Source: CAD feature listing. Evaluate the final solid. Frame: model axes, mm. A direction names the side the tool comes from. Coordinates: 2 decimals unless noted, no trailing zeros. Order: outer loops, then holes, each group sorted by start corner. A loop starts at its lowest first (then second) coordinate and runs counter-clockwise, first axis right, second up. Notation, with made-up numbers: (81.5, 51) - (124.5, 51) arc R20 ccw to (124.5, 68) - close; hole circle Ø7 at (65, 22). An arc over 180 degrees is marked (long way). One line per question, with ' | ' between items. Start each with the question number.
(1) Access query for faces 1 (the flat face through (17.26, 32.27, 22.76)), 2 (the cylindrical face through (16.241, 85.058, -29.11)). Directions: +Z, -Z, +X, -X, +Y, -Y. A direction counts if a zero-diameter tool reaches every point of the face in a straight line with its end or side. Return the directions, or none.
(2) Contact query for flat-ended pins moving along their axis: P1, Ø5, axis at x = 30.5, z = -22, coming from the +Y side; P2, Ø13, axis at y = 22.26, z = 32.96, coming from the -X side; P3, Ø8, axis at x = 16, z = -38.5, coming from the +Y side; P4, Ø9, axis at y = -47.74, z = 32.96, coming from the -X side. Output: stop coordinate, or through.
(3) Section C-C (y = 13.5). Return the cut outline in (x, z).
(4) Section D-D (z = -10.5). Return the cut outline in (x, y).
(5) Section B-B (z = 34.5). Return the cut outline in (x, y).
(6) Draft query along Y for faces 3 (the flat face through (17, -14, 42.956)), 4 (the flat face through (35, 35, 5)), 5 (the flat face through (16.24, 51.94, -0.06)). Return one class per face: +Y half, -Y half, draft (parallel to the pull), parting line (faces both ways), or undercut.
(7) Line query: line 1 along Z through (x, y) = (33.5, 5.5); line 2 along X through (y, z) = (26, 17); line 3 along Y through (x, z) = (3, -10.5). Output: solid intervals per line, ascending.
(8) Section A-A (x = 7.5). Return the cut outline in (y, z).
from build123d import *

# Parameters (mm, degrees)
SKETCH1_R           = 5
BOSS_EXTRUDE1_DEPTH = 2
EXTRUDE_THIN1_DEPTH = 35


# Read off the part's stored shape, not the designer's step: Extrude-Thin1
with BuildPart() as part:
    # Sketch1 → Boss-Extrude1 (new body)
    with BuildSketch(Plane(origin=(0, 0, 0), x_dir=(0, 0, -1), z_dir=(1, 0, 0))):
        with BuildLine():
            Line((49.043932947, -59.7371598), (-44.956067053, -59.7371598))
            Line((-44.956067053, -59.7371598), (-44.956067053, 32.2628402))
            Line((-44.956067053, 32.2628402), (-3.612044261, 36.014733483))
            Line((-3.612044261, 36.014733483), (3.632035406, 67.43070713))
            ThreePointArc((3.632035406, 67.43070713), (28.644544082, 85.115341633), (49.043932947, 62.2628402))
            Line((49.043932947, 62.2628402), (49.043932947, -59.7371598))
        make_face()
        with Locations((37.043932947, 22.2628402)):
            Circle(SKETCH1_R, mode=Mode.SUBTRACT)
        with Locations((37.043932947, -47.7371598)):
            Circle(SKETCH1_R, mode=Mode.SUBTRACT)
        with Locations((-32.956067053, -47.7371598)):
            Circle(SKETCH1_R, mode=Mode.SUBTRACT)
        with Locations((-32.956067053, 22.2628402)):
            Circle(SKETCH1_R, mode=Mode.SUBTRACT)
    extrude(amount=-BOSS_EXTRUDE1_DEPTH)

    # Extrude-Thin1 outline → Extrude-Thin1 (add)
    with BuildSketch(Plane(origin=(0, 0, 0), x_dir=(0, 0, -1), z_dir=(1, 0, 0))):
        with BuildLine():
            Line((-44.956067053, -59.7371598), (49.043932947, -59.7371598))
            Line((49.043932947, -59.7371598), (49.043932947, 62.2628402))
            ThreePointArc((49.043932947, 62.2628402), (28.644544082, 85.115341633), (3.632035406, 67.43070713))
            Line((3.632035406, 67.43070713), (-3.612044261, 36.014733483))
            Line((-3.612044261, 36.014733483), (-44.956067053, 32.2628402))
            Line((-44.956067053, 32.2628402), (-44.956067053, -59.7371598))
        make_face()
        with BuildLine():
            Line((-1.988660061, 34.153834244), (5.255419606, 65.569807891))
            Line((5.255419606, 65.569807891), (7.219966056, 71.571882604))
            ThreePointArc((7.219966056, 71.571882604), (30.82392747, 82.711596944), (47.043932947, 62.2628402))
            Line((47.043932947, 62.2628402), (47.043932947, -57.7371598))
            Line((47.043932947, -57.7371598), (-42.956067053, -57.7371598))
            Line((-42.956067053, -57.7371598), (-42.956067053, 30.436118145))
            Line((-42.956067053, 30.436118145), (-1.988660061, 34.153834244))
        make_face(mode=Mode.SUBTRACT)
    extrude(amount=EXTRUDE_THIN1_DEPTH)


solid = part.part
Response values:
1) face 1: +X | face 2: +X, -X, +Y
2) P1: stops at y = 85.21 | P2: stops at x = -2 | P3: stops at y = 83.65 | P4: passes through
3) outline: (-2, -49.04) - (35, -49.04) - (35, -47.04) - (0, -47.04) - (0, 42.96) - (35, 42.96) - (35, 44.96) - (-2, 44.96) - close
4) outline: (-2, -59.74) - (35, -59.74) - (35, -57.74) - (0, -57.74) - (0, 76.38) - (35, 76.38) - (35, 79.22) - (-2, 79.22) - close
5) outline: (-2, -59.74) - (35, -59.74) - (35, -57.74) - (0, -57.74) - (0, -52.49) - (-2, -52.49) - close; (-2, -42.98) - (0, -42.98) - (0, 17.51) - (-2, 17.51) - close; (-2, 27.02) - (0, 27.02) - (0, 31.2) - (35, 31.2) - (35, 33.21) - (-2, 33.21) - close
6) face 3: undercut | face 4: draft | face 5: +Y half
7) line 1: z = -49.04 to -47.04, 42.96 to 44.96 | line 2: x = -2 to 0 | line 3: y = -59.74 to -57.74, 76.38 to 79.22
8) outline: (-59.74, -49.04) - (62.26, -49.04) arc R23 ccw to (67.43, -3.63) - (36.01, 3.61) - (32.26, 44.96) - (-59.74, 44.96) - close; hole (-57.74, -47.04) - (62.26, -47.04) arc R21 ccw to (71.57, -7.22) - (65.57, -5.26) - (34.15, 1.99) - (30.44, 42.96) - (-57.74, 42.96) - close
